```python
from build123d import *

# Parameters (mm, degrees)
SKETCH1_W               = 78
SKETCH1_H               = 50
KAPTON_INSULATION_DEPTH = 0.127
EDGE_RADIUS_R           = 2.54
SKETCH3_R               = 2.54
MAGNET_HOLE_DEPTH       = 93.649965618
MIRROR2_COPY_1_SKETCH_R = 2.54
MIRROR2_COPY_1_DEPTH    = 93.649965618
SKETCH4_R               = 10.05
CUT_EXTRUDE2_DEPTH      = 93.649965618


with BuildPart() as part:
    # Sketch1 → kapton_insulation (new body)
    with BuildSketch(Plane(origin=(0, 0, 0), x_dir=(1, 0, 0), z_dir=(0, 1, 0))):
        with Locations((39, 25)):
            Rectangle(SKETCH1_W, SKETCH1_H)
    extrude(amount=KAPTON_INSULATION_DEPTH)

    # edge_radius
    edge_radius_edges = [part.edges().sort_by_distance(p)[0] for p in [
        (0, 0.0635, -50),
        (78, 0.0635, -50),
        (78, 0.0635, 0),
        (0, 0.0635, 0),
    ]]
    fillet(edge_radius_edges, radius=EDGE_RADIUS_R)

    # Sketch3 → magnet_hole (cut, through all)
    with BuildSketch(Plane(origin=(0, 0.127, 0), x_dir=(1, 0, 0), z_dir=(0, 1, 0))):
        with Locations(Location((4.1275, 4.1275, 0), (0, 0, 270))):
            Circle(SKETCH3_R)
    magnet_hole = extrude(amount=-MAGNET_HOLE_DEPTH, mode=Mode.SUBTRACT)

    # Mirror1: magnet_hole across plane
    add(magnet_hole.mirror(Plane.XY.offset(-25)), mode=Mode.SUBTRACT)

    # Mirror2: magnet_hole across plane
    add(magnet_hole.mirror(Plane(origin=(39, 0, 0), x_dir=(0, 0, 1), z_dir=(1, 0, 0))), mode=Mode.SUBTRACT)

    # Mirror2 copy 1 sketch → Mirror2 copy 1 (cut, through all)
    with BuildSketch(Plane(origin=(78, 0.127, -50), x_dir=(-1, 0, 0), z_dir=(0, 1, 0))):
        with Locations(Location((4.1275, 4.1275, 0), (0, 0, 270))):
            Circle(MIRROR2_COPY_1_SKETCH_R)
    extrude(amount=-MIRROR2_COPY_1_DEPTH, mode=Mode.SUBTRACT)

    # Sketch4 → Cut-Extrude2 (cut, through all)
    with BuildSketch(Plane(origin=(0, 0.127, 0), x_dir=(1, 0, 0), z_dir=(0, 1, 0))):
        with Locations(Location((61.6, 38.3625, 0), (0, 0, 270))):
            Circle(SKETCH4_R)
        with Locations(Location((39.9125, 38.3625, 0), (0, 0, 270))):
            Circle(SKETCH4_R)
    extrude(amount=-CUT_EXTRUDE2_DEPTH, mode=Mode.SUBTRACT)


solid = part.part
```
For this review, take the finished solid that the model builds, in its own axes (mm). Coordinates: 2 decimals unless noted, no trailing zeros. Write each loop counter-clockwise with the first axis right and the second up, starting at its lowest first coordinate (ties: lowest second). Pieces come first, ordered by that corner, then holes. Notation, with made-up numbers: (-14, 56.5) - (44, 56.5) arc R22 cw to (44, 84.5) - close; hole circle Ø10 at (47, 38.5). An arc over 180 degrees is marked (long way). Answer in a Markdown table with one row per item. Add a question column.
Q1. We need section A-A, the plane x = 61.6. State the section outline as (y, z) points, and give its area (3 significant figures).
Q2. We need section D-D, the plane z = -37.5. State the section outline as (x, y) points.
Q3. For P1, Ø4, axis at x = 73.87, z = -45.87, coming from the +Y side, flat-tipped, find the tip position at first contact; note if it passes through.
Q4. We need section B-B, the plane z = -32. State the section outline as (x, y) points, and give its area (3 significant figures).
Q5. For probe 1 along Z at (x, y) = (3, 0.05); probe 2 along X at (y, z) = (0.05, -46); probe 3 along Z at (x, y) = (36, 0.05), list the stretches that pass through material, from the lowest coordinate up.
Q6. We need section C-C, the plane z = -45. State the section outline as (x, y) points, and give its area (3 significant figures).
Answer list:
| question | item | result |
|---|---|---|
| 1 | outline | (0, -50) - (0.13, -50) - (0.13, -48.41) - (0, -48.41) - close; (0, -28.31) - (0.13, -28.31) - (0.13, 0) - (0, 0) - close |
| 1 | area | 3.80 mm2 |
| 2 | outline | (0, 0) - (29.9, 0) - (29.9, 0.13) - (0, 0.13) - close; (49.93, 0) - (51.59, 0) - (51.59, 0.13) - (49.93, 0.13) - close; (71.61, 0) - (78, 0) - (78, 0.13) - (71.61, 0.13) - close |
| 3 | P1 | passes through |
| 4 | outline | (0, 0) - (32.13, 0) - (32.13, 0.13) - (0, 0.13) - close; (47.69, 0) - (53.82, 0) - (53.82, 0.13) - (47.69, 0.13) - close; (69.38, 0) - (78, 0) - (78, 0.13) - (69.38, 0.13) - close |
| 4 | area | 5.95 mm2 |
| 5 | probe 1 | z = -50 to -48.15, -43.6 to -6.4, -1.85 to 0 |
| 5 | probe 2 | x = 0 to 1.59, 6.66 to 33.38, 46.44 to 55.07, 68.13 to 71.34, 76.41 to 78 |
| 5 | probe 3 | z = -50 to -47.62, -29.11 to 0 |
| 6 | outline | (0, 0) - (1.74, 0) - (1.74, 0.13) - (0, 0.13) - close; (6.51, 0) - (32.37, 0) - (32.37, 0.13) - (6.51, 0.13) - close; (47.46, 0) - (54.05, 0) - (54.05, 0.13) - (47.46, 0.13) - close; (69.15, 0) - (71.49, 0) - (71.49, 0.13) - (69.15, 0.13) - close; (76.26, 0) - (78, 0) - (78, 0.13) - (76.26, 0.13) - close |
| 6 | area | 4.86 mm2 |
